```python
from build123d import *

# Parameters (mm, degrees)
SKETCH1_W               = 60
SKETCH1_H               = 34.3
BOSS_EXTRUDE1_DEPTH     = 6.35
SKETCH2_W               = 15
SKETCH2_H               = 6
BOSS_EXTRUDE2_DEPTH     = 6.35
SKETCH3_R               = 1
CUT_EXTRUDE1_DEPTH      = 7.35
MIRROR2_COPY_1_SKETCH_W = 15
MIRROR2_COPY_1_SKETCH_H = 6
MIRROR2_COPY_1_DEPTH    = 6.35
MIRROR2_COPY_2_SKETCH_R = 1
MIRROR2_COPY_2_DEPTH    = 7.35
FILLET1_R               = 1
FILLET2_R               = 2


with BuildPart() as part:
    # Sketch1 → Boss-Extrude1 (new body)
    with BuildSketch(Plane.XY):
        Rectangle(SKETCH1_W, SKETCH1_H)
    extrude(amount=BOSS_EXTRUDE1_DEPTH)

    # Sketch2 → Boss-Extrude2 (add)
    with BuildSketch(Plane.XY.offset(6.35)):
        with Locations((-17.5, 20.15)):
            Rectangle(SKETCH2_W, SKETCH2_H)
    boss_extrude2 = extrude(amount=-BOSS_EXTRUDE2_DEPTH)

    # Sketch3 → Cut-Extrude1 (cut, through all)
    with BuildSketch(Plane.XY.offset(6.35)):
        with Locations((-25, 17.15)):
            Circle(SKETCH3_R)
        with Locations((-10, 17.15)):
            Circle(SKETCH3_R)
    cut_extrude1 = extrude(amount=-CUT_EXTRUDE1_DEPTH, mode=Mode.SUBTRACT)

    # Mirror1: Boss-Extrude2, Cut-Extrude1 across plane
    add(boss_extrude2.mirror(Plane(origin=(0, 0, 0), x_dir=(0, 0, 1), z_dir=(1, 0, 0))))
    add(cut_extrude1.mirror(Plane(origin=(0, 0, 0), x_dir=(0, 0, 1), z_dir=(1, 0, 0))), mode=Mode.SUBTRACT)

    # Mirror2: Boss-Extrude2, Cut-Extrude1 across plane
    add(boss_extrude2.mirror(Plane.ZX))
    add(cut_extrude1.mirror(Plane.ZX), mode=Mode.SUBTRACT)

    # Mirror2 copy 1 sketch → Mirror2 copy 1 (add)
    with BuildSketch(Plane(origin=(0, 0, 6.35), x_dir=(-1, 0, 0), z_dir=(0, 0, 1))):
        with Locations((-17.5, 20.15)):
            Rectangle(MIRROR2_COPY_1_SKETCH_W, MIRROR2_COPY_1_SKETCH_H)
    extrude(amount=-MIRROR2_COPY_1_DEPTH)

    # Mirror2 copy 2 sketch → Mirror2 copy 2 (cut, through all)
    with BuildSketch(Plane(origin=(0, 0, 6.35), x_dir=(-1, 0, 0), z_dir=(0, 0, 1))):
        with Locations((-25, 17.15)):
            Circle(MIRROR2_COPY_2_SKETCH_R)
        with Locations((-10, 17.15)):
            Circle(MIRROR2_COPY_2_SKETCH_R)
    extrude(amount=-MIRROR2_COPY_2_DEPTH, mode=Mode.SUBTRACT)

    # Fillet1
    fillet1_edges = [part.edges().sort_by_distance(p)[0] for p in [
        (26, -17.15, 3.175),
        (9, -17.15, 3.175),
        (-10, -23.15, 3.175),
        (-25, -23.15, 3.175),
        (-25, -18.15, 3.175),
        (-10, -18.15, 3.175),
        (-26, -17.15, 3.175),
        (-9, -17.15, 3.175),
        (-25, 23.15, 3.175),
        (-10, 23.15, 3.175),
        (-10, 18.15, 3.175),
        (-25, 18.15, 3.175),
        (-26, 17.15, 3.175),
        (-9, 17.15, 3.175),
        (10, 23.15, 3.175),
        (25, 23.15, 3.175),
        (25, 18.15, 3.175),
        (10, 18.15, 3.175),
        (26, 17.15, 3.175),
        (9, 17.15, 3.175),
        (25, -23.15, 3.175),
        (10, -23.15, 3.175),
        (10, -18.15, 3.175),
        (25, -18.15, 3.175),
    ]]
    fillet(fillet1_edges, radius=FILLET1_R)

    # Fillet2
    fillet2_edges = [part.edges().sort_by_distance(p)[0] for p in [
        (-30, 17.15, 3.175),
        (30, 17.15, 3.175),
        (30, -17.15, 3.175),
        (-30, -17.15, 3.175),
    ]]
    fillet(fillet2_edges, radius=FILLET2_R)


solid = part.part
```
Check sheet for the modelled part. Datum: model origin and axes. Units: mm. A direction names the side the tool comes from. Coordinates: 2 decimals unless noted, no trailing zeros. Order: outer loops, then holes, each group sorted by start corner. A loop starts at its lowest first (then second) coordinate and runs counter-clockwise, first axis right, second up. Notation, with made-up numbers: M 89,89.5 L 134,89.5 A18 cw 134,97.5 Z; hole C 41,72.25 d4. An arc over 180 degrees is marked long. Write each question's results on one line, items separated by ' | '. Start each with the question number.
1. Material ranges on probe 1 along X at (y, z) = (20.5, 5.5); probe 2 along Y at (x, z) = (0.5, 3); probe 3 along X at (y, z) = (18, 3), recorded low to high.
2. Mould release check, pull along X, two halves, no side actions. Record for faces 1 (the face through (-27, -17.15, 3)), 2 (the face through (-25, 20, 3)), 3 (the face through (-10, 20, 3)): +X half, -X half, draft (parallel to the pull), parting line (faces both ways), or undercut.
3. Cross-section at A-A on x = 4. Record the cut outline in (y, z).
4. Access from +Z, -Z, +X, -X, +Y, -Y to the whole of each face (thin tool, end or side, straight path). Record for faces 4 (the face through (27, -17.15, 3)), 5 (the face through (0, -17.15, 3)), 6 (the face through (0, 17.15, 3)), 7 (the face through (25, 20, 3)).
5. Go/stop test with flat-tipped pins: P1, Ø1.9, axis at x = 4, z = 2, coming from the -Y side; P2, Ø1.6, axis at y = -21, z = 4.5, coming from the -X side; P3, Ø1, axis at y = -20.5, z = 3, coming from the +X side. Record where each tip stops, or that it passes through.
Checks:
1) probe 1: x = -25 to -10, 10 to 25 | probe 2: y = -17.15 to 17.15 | probe 3: x = -24.47 to -10.53, 10.53 to 24.47
2) face 1: draft | face 2: -X half | face 3: undercut
3) outline: M -17.15,0 L 17.15,0 L 17.15,6.35 L -17.15,6.35 Z
4) face 4: +Z, -Z, +X, -Y | face 5: +Z, -Z, -Y | face 6: +Z, -Z, +Y | face 7: +Z, -Z, +X, +Y
5) P1: stops at y = -17.15 | P2: stops at x = -25 | P3: stops at x = 25
